For this review, take the finished solid that the model builds, in its own axes (mm). A direction names the side the tool comes from. Give positions to 0.01 mm unless a question says otherwise; leave off trailing zeros. Order: outer loops, then holes, each group sorted by start corner. A loop starts at its lowest first (then second) coordinate and runs counter-clockwise, first axis right, second up. Notation, with made-up numbers: (59.5, 8) - (114.5, 8) arc R9 ccw to (114.5, 25) - close; hole circle Ø10 at (18, -7.5). An arc over 180 degrees is marked (long way). Use a Markdown table: item, result. Add a question column.
1) We need section A-A on z = 3.5. Write out the cut boundary in (x, y), then the cut area to 3 significant figures.
2) Wall thickness on L1, parallel to Y at x = -19, z = 3.75; L2, parallel to Y at x = 4.5, z = 6.5; L3, parallel to X at y = 58, z = 18: over which ranges is each line inside the solid? List them lowest first.
3) We need section B-B on x = 4. Write out the cut boundary in (y, z), then the cut area to 3 significant figures.
4) Clearance check with a flat-ended pin moving along its axis: P1, Ø6, axis at x = 35, z = 17, coming from the +Y side. State where the tip first meets the part, or that it passes through.
5) We need section C-C on y = 51.5. Write out the cut boundary in (x, z), then the cut area to 3 significant figures.
6) Mouldability with a two-part tool opening along Y and no side actions: class faces 1 (the face through (0, 0, 13)), 2 (the face through (-1.645, 46.645, 12.878)), 3 (the face through (45.37, 70.47, 12.88)) as released by +Y, released by -Y, zero draft, split by the parting line, or undercut.
7) We need section D-D on x = 39. Write out the cut boundary in (y, z).
8) Machinability: for faces 4 (the face through (0, 76.2, 13)), 5 (the face through (-2.143, 33.932, 12.878)), which of the approach directions +Z, -Z, +X, -X, +Y, -Y give a long, thin tool a straight path to every point of the face, cutting with its end or side? Answer none if there is none.
```python
from build123d import *

# Parameters (mm, degrees)
F1_DEPTH = 25.4
F2_R     = 19.05
F4_DEPTH = 254


with BuildPart() as f1:
    # F0 (on Top) → F1 (new body)
    with BuildSketch(Plane.XY):
        Polygon((-50.8, 0), (0, 0), (50.8, 0), (50.8, 76.2), (-50.8, 76.2), align=None)
    extrude(amount=F1_DEPTH)

    # F2
    f2_edges = [f1.edges().sort_by_distance(p)[0] for p in [
        (-50.8, 0, 12.7),
        (50.8, 0, 12.7),
        (-50.8, 76.2, 12.7),
        (50.8, 76.2, 12.7),
    ]]
    fillet(f2_edges, radius=F2_R)

    # F3 (on face) → F4 (cut)
    with BuildSketch(Plane.XY.offset(25.4)):
        Polygon((-19.6837, 52.613977), (-19.6837, 27.213977), (15.896244, 40.840335), align=None)
    extrude(amount=-F4_DEPTH, mode=Mode.SUBTRACT)


solid = f1.part
```
Checked values:
| question | item | result |
|---|---|---|
| 1 | outline | (-50.8, 19.05) arc R19.05 ccw to (-31.75, 0) - (31.75, 0) arc R19.05 ccw to (50.8, 19.05) - (50.8, 57.15) arc R19.05 ccw to (31.75, 76.2) - (-31.75, 76.2) arc R19.05 ccw to (-50.8, 57.15) - close; hole (-19.68, 27.21) - (15.9, 40.84) - (-19.68, 52.61) - close |
| 1 | area | 6,980 mm² |
| 2 | L1 | 0 to 27.48, 52.39 to 76.2 |
| 2 | L2 | 0 to 36.48, 44.61 to 76.2 |
| 2 | L3 | -50.78 to 50.78 |
| 3 | outline | (0, 0) - (36.28, 0) - (36.28, 25.4) - (0, 25.4) - close; (44.78, 0) - (76.2, 0) - (76.2, 25.4) - (44.78, 25.4) - close |
| 3 | area | 1,720 mm² |
| 4 | P1 | y = 76.2 |
| 5 | outline | (-50.8, 0) - (-19.68, 0) - (-19.68, 25.4) - (-50.8, 25.4) - close; (-16.32, 0) - (50.8, 0) - (50.8, 25.4) - (-16.32, 25.4) - close |
| 5 | area | 2,500 mm² |
| 6 | face 1 | released by -Y |
| 6 | face 2 | undercut |
| 6 | face 3 | released by +Y |
| 7 | outline | (1.43, 0) - (74.77, 0) - (74.77, 25.4) - (1.43, 25.4) - close |
| 8 | face 4 | +Z, -Z, +X, -X, +Y |
| 8 | face 5 | +Z, -Z |
